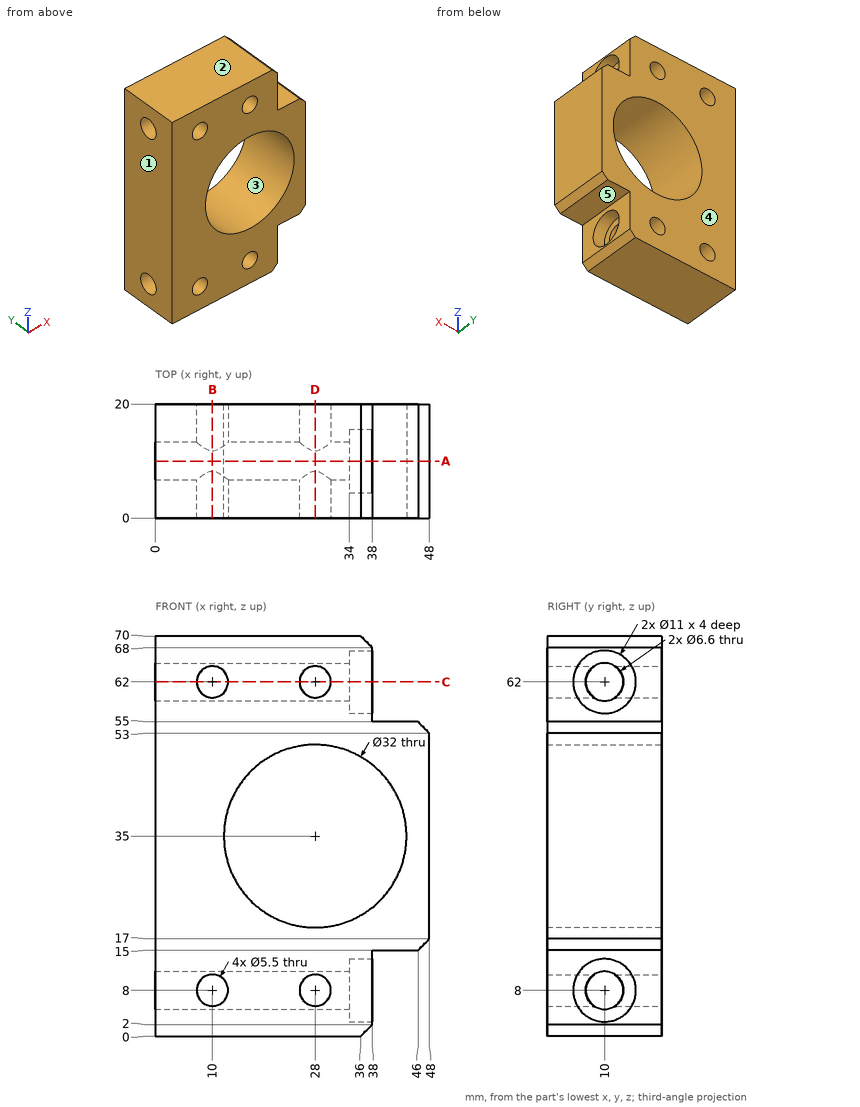
Job drawing, mm, ordinate dimensions from the low corner. One solid piece. A direction names the side the tool comes from. Round coordinates to 2 decimals unless told otherwise and drop trailing zeros. Loops run counter-clockwise (first coordinate to the right, second up) from the corner with the lowest first, then second, coordinate; pieces in that order, holes last.
(1) Cut at B-B (x = 10). Give the cut face in (y, z).
(2) Cut at C-C (z = 62). Give the cut face in (x, y), plus the area to 3 significant figures.
(3) Wall check: line 1 along Z through (x, y) = (10, 6.25); line 2 along Z through (x, y) = (28, 15); line 3 along Z through (x, y) = (28, 10). Give the ranges that are in metal, low to high.
(4) Cut at A-A (y = 10). State how many separate pieces and enclosed holes the cut face has, plus the area to 3 significant figures.
(5) Two-plate mould, pull along Z, no slides. Class the marked faces 1, 2 and 3: +Z half, -Z half, draft (parallel to the pull), parting line (faces both ways), or undercut.
(6) Drop flat-ended pins along their axis: pin 1 (6.5 mm diameter, centred on x = 44, y = 9, fed in from +Z); pin 2 (9 mm diameter, centred on y = 12.5, z = 6, fed in from +X); pin 3 (5 mm diameter, centred on x = 41.5, y = 14.5, fed in from -Z). Give the stop position or say it passes through.
(7) Which spindle directions (+Z, -Z, +X, -X, +Y, -Y) get a long thin tool onto all of the face, cutting with end or side? Do the marked faces 4 and 5. Say none if no direction does.
(8) Cut at D-D (x = 28). Give the cut face in (y, z), plus the area to 3 significant figures.
Findings below:
1. outline: (0, 0) - (20, 0) - (20, 5.25) - (11.82, 5.25) arc R3.3 cw to (8.18, 5.25) - (0, 5.25) - close; (0, 10.75) - (8.18, 10.75) arc R3.3 cw to (11.82, 10.75) - (20, 10.75) - (20, 59.25) - (11.82, 59.25) arc R3.3 cw to (8.18, 59.25) - (0, 59.25) - close; (0, 64.75) - (8.18, 64.75) arc R3.3 cw to (11.82, 64.75) - (20, 64.75) - (20, 70) - (0, 70) - close
2. outline: (0, 0) - (7.25, 0) - (7.25, 6.7) - (0, 6.7) - close; (0, 13.3) - (7.25, 13.3) - (7.25, 20) - (0, 20) - close; (12.75, 0) - (25.25, 0) - (25.25, 6.7) - (12.75, 6.7) - close; (12.75, 13.3) - (25.25, 13.3) - (25.25, 20) - (12.75, 20) - close; (30.75, 0) - (38, 0) - (38, 4.5) - (34, 4.5) - (34, 6.7) - (30.75, 6.7) - close; (30.75, 13.3) - (34, 13.3) - (34, 15.5) - (38, 15.5) - (38, 20) - (30.75, 20) - close
2. area: 344 mm2
3. line 1: z = 0 to 5.25, 10.75 to 59.25, 64.75 to 70
3. line 2: z = 0 to 5.25, 10.75 to 19, 51 to 59.25, 64.75 to 70
3. line 3: z = 0 to 4.7, 11.3 to 19, 51 to 58.7, 65.3 to 70
4. separate pieces: 3
4. enclosed holes: 1
4. area: 1,710 mm2
5. face 1: draft
5. face 2: +Z half
5. face 3: undercut
6. pin 1: stops at z = 55
6. pin 2: stops at x = 38
6. pin 3: stops at z = 15
7. face 4: +Z, -Z, +X, -X, +Y
7. face 5: -Z, +X, +Y, -Y
8. outline: (0, 0) - (20, 0) - (20, 5.25) - (11.82, 5.25) arc R3.3 cw to (8.18, 5.25) - (0, 5.25) - close; (0, 10.75) - (8.18, 10.75) arc R3.3 cw to (11.82, 10.75) - (20, 10.75) - (20, 19) - (0, 19) - close; (0, 51) - (20, 51) - (20, 59.25) - (11.82, 59.25) arc R3.3 cw to (8.18, 59.25) - (0, 59.25) - close; (0, 64.75) - (8.18, 64.75) arc R3.3 cw to (11.82, 64.75) - (20, 64.75) - (20, 70) - (0, 70) - close
8. area: 535 mm2
